Input: part model. Units: mm. Frame: model coordinates. A direction names the side the tool comes from. Give positions to 0.01 mm unless a question says otherwise; leave off trailing zeros. Loops run counter-clockwise (first coordinate to the right, second up) from the corner with the lowest first, then second, coordinate; pieces in that order, holes last. Notation, with made-up numbers: (29.5, 50.5) - (85.5, 50.5) arc R23 ccw to (85.5, 71.5) - close; hole circle Ø7 at (28, 4). An arc over 180 degrees is marked (long way). Answer as a JSON object with one key per item and string values. Group by question number.
(1) Section query B-B (y = 643.5). Return loops of the section in (x, z).
(2) Section query C-C (z = 1578.2). Count the separate pieces of the cut face and the enclosed holes in it, plus the area to 3 significant figures.
(3) Section query D-D (y = 658). Return loops of the section in (x, z).
(4) Section query A-A (x = 250). Return loops of the section in (y, z).
(5) Material intervals for L1, parallel to X at y = 669.5, z = 1578.6; L2, parallel to X at y = 636, z = 1579.5; L3, parallel to Y at x = 242, z = 1579, sorted ascending.
(6) Pin query (flat end, axial travel): P1, Ø6.5, axis at x = 226.78, y = 617.2, coming from the +Z side; P2, Ø1.5, axis at x = 227.5, z = 1579, coming from the +Y side; P3, Ø1.5, axis at y = 657.5, z = 1578.5, coming from the -X side. Return the tip coordinate at first contact, or that it passes through.
(7) Access query for faces 1 (the cylindrical face through (271.446, 657.646, 1579.24)), 2 (the flat face through (261.432, 633.135, 1579.195)), 3 (the flat face through (215.564, 654.506, 1579.195)). Directions: +Z, -Z, +X, -X, +Y, -Y. A direction counts if a zero-diameter tool reaches every point of the face in a straight line with its end or side. Return the directions, or none.
```python
from build123d import *

# Parameters (mm, degrees)
BOSS_EXTRUDE1_DEPTH  = 3.175
SKETCH1_4_R          = 4
SKETCH1_4_R_2        = 3.175
HOLES_DEPTH          = 3.175
SKETCH5_OUTSIDE_W    = 151.471
SKETCH5_OUTSIDE_H    = 153.323
OUTSIDEEXTRUDE_DEPTH = 3.81
INNERTRIANGLE_DEPTH  = 3.81
FILLET2_R            = 6.35
FILLET3_R            = 2.54


with BuildPart() as part:
    # Sketch1 → Boss-Extrude1 (new body)
    with BuildSketch(Plane.XY.offset(1577.629912845)):
        Polygon((200.232199361, 713.672399287), (217.036775663, 595.514826781), (316.536854979, 661.418847479), align=None)
    extrude(amount=BOSS_EXTRUDE1_DEPTH)

    # Sketch1<4> → Holes (cut)
    with BuildSketch(Plane.XY.offset(1577.629912845)):
        with Locations((216.050914922, 692.642443937)):
            Circle(SKETCH1_4_R)
        with Locations((290.308718483, 659.279772728)):
            Circle(SKETCH1_4_R_2)
        with Locations((226.780244033, 617.20159627)):
            Circle(SKETCH1_4_R)
    extrude(amount=HOLES_DEPTH, mode=Mode.SUBTRACT)

    # Sketch5 outside → OutsideExtrude (cut)
    with BuildSketch(Plane(origin=(0, 0, 1577.629912845), x_dir=(-1, 0, 0), z_dir=(0, 0, -1))):
        with Locations((-258.3845, 654.5935)):
            Rectangle(SKETCH5_OUTSIDE_W, SKETCH5_OUTSIDE_H)
        with BuildLine():
            Line((-211.315771723, 684.377817887), (-219.928647009, 623.818335891))
            ThreePointArc((-219.928647009, 623.818335891), (-222.876711188, 608.51320998), (-236.277349403, 616.473163308))
            Line((-236.277349403, 616.473163308), (-287.274277772, 650.251052189))
            ThreePointArc((-287.274277772, 650.251052189), (-299.802198055, 660.0540276), (-285.851407356, 667.697492284))
            Line((-285.851407356, 667.697492284), (-225.304484054, 694.900116089))
            ThreePointArc((-225.304484054, 694.900116089), (-210.325206852, 700.25440111), (-211.315771723, 684.377817887))
        make_face(mode=Mode.SUBTRACT)
    extrude(amount=-OUTSIDEEXTRUDE_DEPTH, mode=Mode.SUBTRACT)

    # Sketch6 → InnerTriangle (cut)
    with BuildSketch(Plane(origin=(0, 0, 1577.629912845), x_dir=(-1, 0, 0), z_dir=(0, 0, -1))):
        Polygon((-223.339566396, 682.952655016), (-231.269656883, 627.194019699), (-278.223809028, 658.294169931), align=None)
    extrude(amount=-INNERTRIANGLE_DEPTH, mode=Mode.SUBTRACT)

    # Fillet2
    fillet2_edges = [part.edges().sort_by_distance(p)[0] for p in [
        (278.223809028, 658.294169931, 1579.217412845),
        (223.339566396, 682.952655016, 1579.217412845),
        (231.269656883, 627.194019699, 1579.217412845),
    ]]
    fillet(fillet2_edges, radius=FILLET2_R)

    # Fillet3
    fillet3_edges = [part.edges().sort_by_distance(p)[0] for p in [
        (211.315771723, 684.377817887, 1579.217412845),
        (219.928647009, 623.818335891, 1579.217412845),
        (236.277349403, 616.473163308, 1579.217412845),
        (287.274277772, 650.251052189, 1579.217412845),
        (285.851407356, 667.697492284, 1579.217412845),
        (225.304484054, 694.900116089, 1579.217412845),
    ]]
    fillet(fillet3_edges, radius=FILLET3_R)


solid = part.part
```
Recorded:
{
 "1": {"outline": "(217.13, 1577.63) - (228.95, 1577.63) - (228.95, 1580.8) - (217.13, 1580.8) - close; (255.89, 1577.63) - (277.08, 1577.63) - (277.08, 1580.8) - (255.89, 1580.8) - close"},
 "2": {"separate pieces": "1", "enclosed holes": "4", "area": "2,910 mm^2"},
 "3": {"outline": "(215.07, 1577.63) - (226.89, 1577.63) - (226.89, 1580.8) - (215.07, 1580.8) - close; (271.41, 1577.63) - (287.4, 1577.63) - (287.4, 1580.8) - (271.41, 1580.8) - close; (293.21, 1577.63) - (299.75, 1577.63) - (299.75, 1580.8) - (293.21, 1580.8) - close"},
 "4": {"outline": "(625.56, 1577.63) - (639.6, 1577.63) - (639.6, 1580.8) - (625.56, 1580.8) - close; (670.97, 1577.63) - (683.8, 1577.63) - (683.8, 1580.8) - (670.97, 1580.8) - close"},
 "5": {"L1": "x = 213.43 to 225.25, 253.28 to 281.84", "L2": "x = 218.2 to 230.13, 244.56 to 265.76", "L3": "y = 620.26 to 634.3, 674.57 to 687.4"},
 "6": {"P1": "passes through", "P2": "stops at y = 694.25", "P3": "stops at x = 215.03"},
 "7": {"face 1": "+Z, -Z", "face 2": "+Z, -Z, +X, -Y", "face 3": "+Z, -Z, -X"}
}
